Read the model definition and answer for the solid it produces. Units are mm, in the model's axes. Face numbers are marked on the shaded views. A direction names the side the tool comes from. Give positions to 0.01 mm unless a question says otherwise; leave off trailing zeros. Order: outer loops, then holes, each group sorted by start corner. A loop starts at its lowest first (then second) coordinate and runs counter-clockwise, first axis right, second up. Notation, with made-up numbers: (-39.75, 1.5) - (19.25, 1.5) arc R30 ccw to (19.25, 37.5) - close; hole circle Ø6 at (8, 40.5). An arc over 180 degrees is marked (long way). Return JSON: item names as keys, results as strings.
```python
from build123d import *

# Parameters (mm, degrees)
SKETCH4_R                  = 2
SKETCH4_R_2                = 0.9525
BOSS_EXTRUDE1_DEPTH        = 1.4
BOSS_EXTRUDE1_2_DEPTH      = 1.4
SKETCH5_R                  = 0.9271
BOSS_EXTRUDE2_DEPTH        = 0.6096
LPATTERN1_COUNT            = 2
LPATTERN1_PITCH            = 5.9944
SKETCH7_R                  = 0.9271
BOSS_EXTRUDE3_DEPTH        = 0.6096
BOSS_EXTRUDE4_DEPTH        = 4.1402
BOSS_EXTRUDE4_DEPTH_BACK   = 4.1402
SKETCH8_R                  = 0.9271
BOSS_EXTRUDE4_2_DEPTH      = 4.1402
BOSS_EXTRUDE4_2_DEPTH_BACK = 4.1402
LPATTERN2_COUNT            = 2
LPATTERN2_PITCH            = 11.9888


with BuildPart() as part:
    # Sketch4 → Boss-Extrude1 (new, symmetric)
    with BuildSketch(Plane.XY):
        with Locations((-2.9972, 0)):
            Circle(SKETCH4_R)
        with Locations((-2.9972, 0)):
            Circle(SKETCH4_R_2, mode=Mode.SUBTRACT)
    extrude(amount=BOSS_EXTRUDE1_DEPTH, both=True)


with BuildPart() as body_2:
    # Sketch4 → Boss-Extrude1 2 (new, symmetric)
    with BuildSketch(Plane.XY):
        with Locations((2.9972, 0)):
            Circle(SKETCH4_R)
        with Locations((2.9972, 0)):
            Circle(SKETCH4_R_2, mode=Mode.SUBTRACT)
    extrude(amount=BOSS_EXTRUDE1_2_DEPTH, both=True)


with BuildPart() as body_3:
    # Sketch5 → Boss-Extrude2 (new body)
    with BuildSketch(Plane.XY.offset(1.4)):
        with BuildLine():
            ThreePointArc((-2.380336072, 2.424661318), (-5.4991, 0), (-2.380336072, -2.424661318))
            ThreePointArc((-2.380336072, -2.424661318), (0, -2.126615), (2.380336072, -2.424661318))
            ThreePointArc((2.380336072, -2.424661318), (5.4991, 0), (2.380336072, 2.424661318))
            ThreePointArc((2.380336072, 2.424661318), (0, 2.126615), (-2.380336072, 2.424661318))
        make_face()
        with Locations((-2.9972, 0)):
            Circle(SKETCH5_R, mode=Mode.SUBTRACT)
        with Locations((2.9972, 0)):
            Circle(SKETCH5_R, mode=Mode.SUBTRACT)
    extrude(amount=BOSS_EXTRUDE2_DEPTH)


with BuildPart() as lpattern1_1:
    # LPattern1: pattern copy
    add(body_2.part.moved(Location(Vector(1, 0, 0) * (1 * LPATTERN1_PITCH))))


with BuildPart() as body_5:
    # Sketch7 → Boss-Extrude3 (new body)
    with BuildSketch(Plane.XY.offset(-2.0604)):
        with BuildLine():
            ThreePointArc((3.553786614, 2.130157491), (0.795528, 0), (3.553786614, -2.130157491))
            ThreePointArc((3.553786614, -2.130157491), (5.9944, -1.816568799), (8.435013386, -2.130157491))
            ThreePointArc((8.435013386, -2.130157491), (11.193272, 0), (8.435013386, 2.130157491))
            ThreePointArc((8.435013386, 2.130157491), (5.9944, 1.816568799), (3.553786614, 2.130157491))
        make_face()
        with Locations((2.9972, 0)):
            Circle(SKETCH7_R, mode=Mode.SUBTRACT)
        with Locations((8.9916, 0)):
            Circle(SKETCH7_R, mode=Mode.SUBTRACT)
    extrude(amount=-BOSS_EXTRUDE3_DEPTH)


with BuildPart() as body_6:
    # Mirror1: mirrored copy
    add(body_3.part.mirror(Plane.XY))


with BuildPart() as body_7:
    # Mirror1 2: mirrored copy
    add(body_5.part.mirror(Plane.XY))


with BuildPart() as body_8:
    # Sketch8 → Boss-Extrude4 (new, two sides: drawn at the far end of the back side and taken through both)
    with BuildSketch(Plane.XY.offset(-BOSS_EXTRUDE4_DEPTH_BACK)):
        with Locations((2.9972, 0)):
            Circle(SKETCH8_R)
    extrude(amount=BOSS_EXTRUDE4_DEPTH + BOSS_EXTRUDE4_DEPTH_BACK)


with BuildPart() as body_9:
    # Sketch8 → Boss-Extrude4 2 (new, two sides: drawn at the far end of the back side and taken through both)
    with BuildSketch(Plane.XY.offset(-BOSS_EXTRUDE4_2_DEPTH_BACK)):
        with Locations((8.9916, 0)):
            Circle(SKETCH8_R)
    extrude(amount=BOSS_EXTRUDE4_2_DEPTH + BOSS_EXTRUDE4_2_DEPTH_BACK)


with BuildPart() as lpattern2_1:
    # LPattern2: pattern copy
    add(body_9.part.moved(Location(Vector(1, 0, 0) * (1 * LPATTERN2_PITCH))))


with BuildPart() as lpattern2_2:
    # LPattern2: pattern copy
    add(body_8.part.moved(Location(Vector(1, 0, 0) * (1 * LPATTERN2_PITCH))))


with BuildPart() as lpattern2_3:
    # LPattern2: pattern copy
    add(body_7.part.moved(Location(Vector(1, 0, 0) * (1 * LPATTERN2_PITCH))))


with BuildPart() as lpattern2_4:
    # LPattern2: pattern copy
    add(body_6.part.moved(Location(Vector(1, 0, 0) * (1 * LPATTERN2_PITCH))))


with BuildPart() as lpattern2_5:
    # LPattern2: pattern copy
    add(body_5.part.moved(Location(Vector(1, 0, 0) * (1 * LPATTERN2_PITCH))))


with BuildPart() as lpattern2_6:
    # LPattern2: pattern copy
    add(lpattern1_1.part.moved(Location(Vector(1, 0, 0) * (1 * LPATTERN2_PITCH))))


with BuildPart() as lpattern2_7:
    # LPattern2: pattern copy
    add(body_3.part.moved(Location(Vector(1, 0, 0) * (1 * LPATTERN2_PITCH))))


with BuildPart() as lpattern2_8:
    # LPattern2: pattern copy
    add(body_2.part.moved(Location(Vector(1, 0, 0) * (1 * LPATTERN2_PITCH))))


with BuildPart() as lpattern2_9:
    # LPattern2: pattern copy
    add(part.part.moved(Location(Vector(1, 0, 0) * (1 * LPATTERN2_PITCH))))


with BuildPart() as body_2_1:
    add(body_2.part)

    # Combine1: union body 3, LPattern1_1, body 5, body 6, body 7, body 8, body 9, LPattern2_1, LPattern2_2, LPattern2_3, LPattern2_4, LPattern2_5, LPattern2_7, LPattern2_8, LPattern2_9, part
    add(body_3.part)
    add(lpattern1_1.part)
    add(body_5.part)
    add(body_6.part)
    add(body_7.part)
    add(body_8.part)
    add(body_9.part)
    add(lpattern2_1.part)
    add(lpattern2_2.part)
    add(lpattern2_3.part)
    add(lpattern2_4.part)
    add(lpattern2_5.part)
    add(lpattern2_7.part)
    add(lpattern2_8.part)
    add(lpattern2_9.part)
    add(part.part)


solid = body_2_1.part
```
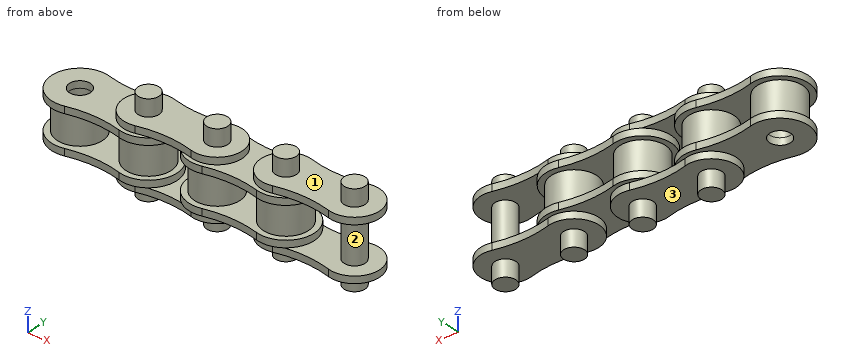
Q1. For the marked faces 1, 2 and 3, determine the directions among +Z, -Z, +X, -X, +Y, -Y from which every point of the face is accessible in a straight line to the end or side of a thin tool.
Values:
{"face 1": "+Z", "face 2": "none", "face 3": "-Z"}
Q2. A cutting plane is placed at B-B (y = 0). Give the number of separate pieces and of enclosed holes in the cut face, and give its area (3 significant figures).
Values:
{"separate pieces": "2", "enclosed holes": "10", "area": "119 mm²"}
Q3. A cutting plane is placed at A-A (z = -1.75). Write down the section's boundary in (x, y), and give its area (3 significant figures).
Values:
{"outline": "(-2.38, -2.42) arc R9.65 cw to (2.38, -2.42) arc R2.5 ccw (long way) to (2.38, 2.42) arc R9.65 cw to (-2.38, 2.42) arc R2.5 ccw (long way) to start; (9.61, -2.42) arc R9.65 cw to (14.37, -2.42) arc R2.5 ccw (long way) to (14.37, 2.42) arc R9.65 cw to (9.61, 2.42) arc R2.5 ccw (long way) to start; circle Ø1.85 at (20.98, 0); hole circle Ø1.85 at (-3, 0)", "area": "93.9 mm²"}
Q4. Given pin 1 (1.5 mm diameter, centred on x = 5, y = 1.5, fed in from -Z); pin 2 (1 mm diameter, centred on x = -2.5, y = -0.5, fed in from +Z); pin 3 (1 mm diameter, centred on x = 10.5, z = -1, fed in from -Y); pin 4 (2 mm diameter, centred on x = 20, y = 0, fed in from -Z), each flat-ended and moving along its own axis, determine where each tip first touches the part or whether it passes through.
Values:
{"pin 1": "stops at z = -2.67", "pin 2": "stops at z = 2.01", "pin 3": "stops at y = -2.29", "pin 4": "stops at z = -4.14"}
Q5. Consider L1, parallel to Z at x = 12.75, y = 1.4; L2, parallel to Z at x = 19.5, y = 1.65; L3, parallel to X at y = 1.2, z = 0.75. Determine where each line is inside the solid, lowest interval first.
Values:
{"L1": "z = -2.01 to -1.4, 1.4 to 2.01", "L2": "z = -2.67 to -2.06, 2.06 to 2.67", "L3": "x = -4.6 to -1.4, 1.4 to 4.6, 7.39 to 10.59, 13.39 to 16.59"}
Q6. A cutting plane is placed at C-C (x = 1.75). Write down the section's boundary in (y, z), and give its area (3 significant figures).
Values:
{"outline": "(-2.29, -2.01) - (2.29, -2.01) - (2.29, -1.4) - (1.56, -1.4) - (1.56, 1.4) - (2.29, 1.4) - (2.29, 2.01) - (-2.29, 2.01) - (-2.29, 1.4) - (-1.56, 1.4) - (-1.56, -1.4) - (-2.29, -1.4) - close; (-1.81, -2.67) - (1.81, -2.67) - (1.81, -2.06) - (-1.81, -2.06) - close; (-1.81, 2.06) - (1.81, 2.06) - (1.81, 2.67) - (-1.81, 2.67) - close", "area": "18.8 mm²"}
